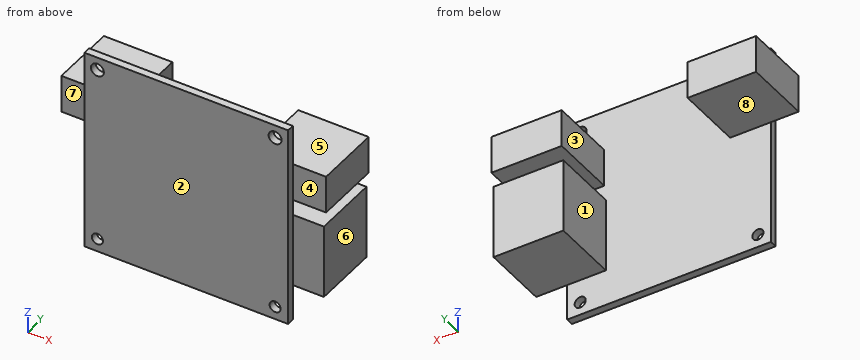
Autodesk Inventor part; units mm, degrees
ref_plane "YZ Plane" through (0, 0, 0) normal (1, 0, 0) x (0, 1, 0)
ref_plane "XZ Plane" through (0, 0, 0) normal (0, 1, 0) x (-1, 0, 0)
ref_plane "XY Plane" through (0, 0, 0) normal (0, 0, 1) x (1, 0, 0)
sketch "Sketch1" plane through (0, 0, 0) normal (0, 1, 0) x (-1, 0, 0)
  line L0 (0, 0) -> (-55, 0)
  line L1 (-55, 0) -> (-55, -55)
  line L2 (-55, -55) -> (0, -55)
  line L3 (0, -55) -> (0, 0)
  circle A0 centre (-3.5, -51.5) radius 1.5
  circle A1 centre (-51.5, -51.5) radius 1.5
  circle A2 centre (-3.5, -3.5) radius 1.75
  circle A3 centre (-51.5, -3.5) radius 1.75
  line L4 (-80.9711, 26.8887) -> (29.0289, 26.8887) construction
  line L5 (29.0289, 26.8887) -> (29.0289, -83.1113) construction
  line L6 (29.0289, -83.1113) -> (-80.9711, -83.1113) construction
  line L7 (-80.9711, -83.1113) -> (-80.9711, 26.8887) construction
  dimension "d1" = 55
  dimension "d4" = 55
  dimension "d49" = 3.5
  dimension "d50" = 3.5
  dimension "d51" = 3
  dimension "d54" = 3
  dimension "d55" = 3.5
  dimension "d56" = 3.5
  dimension "d59" = 3.5
  dimension "d60" = 3.5
  dimension "d61" = 3.5
  dimension "d62" = 3.5
  dimension "d63" = 3.5
  dimension "d64" = 3.5
  dimension "d90" = 110
extrude "Extrusion1" add sketch "Sketch1" along normal blind 2
sketch "Sketch4" plane through (0, 2, 0) normal (0, 1, 0) x (1, 0, 0)
  line L0 (-26.0558, 81.8781) -> (83.9442, 81.8781) construction
  line L1 (83.9442, 81.8781) -> (83.9442, -28.1219) construction
  line L2 (83.9442, -28.1219) -> (-26.0558, -28.1219) construction
  line L3 (-26.0558, -28.1219) -> (-26.0558, 81.8781) construction
  point P0 (0, 0)
  dimension "d77" = 110
sketch "Sketch5" plane through (0, 2, 0) normal (0, 1, 0) x (1, 0, 0)
  line L0 (44.5715, 45.2054) -> (63.4108, 45.2054)
  line L1 (63.4108, 45.2054) -> (63.4108, 25.2259)
  line L2 (63.4108, 25.2259) -> (44.5715, 25.2259)
  line L3 (44.5715, 25.2259) -> (44.5715, 45.2054)
  line L4 (45, 21) -> (64, 21)
  line L5 (64, 21) -> (64, 10.8389)
  line L6 (64, 10.8389) -> (45, 10.8389)
  line L7 (45, 10.8389) -> (45, 21)
  line L8 (-7.4993, 21) -> (11, 21)
  line L9 (11, 21) -> (11, 10.8389)
  line L10 (11, 10.8389) -> (-7.4993, 10.8389)
  line L11 (-7.4993, 10.8389) -> (-7.4993, 21)
  point P0 (0, 0)
extrude "Extrusion2" add sketch "Sketch5" along normal blind 18
properties part number "motorcontroller"
Input: part model. Units: mm. Frame: model coordinates. Face numbers are marked on the shaded views. A direction names the side the tool comes from. Give positions to 0.01 mm unless a question says otherwise; leave off trailing zeros. Order: outer loops, then holes, each group sorted by start corner. A loop starts at its lowest first (then second) coordinate and runs counter-clockwise, first axis right, second up. Notation, with made-up numbers: (15.5, 52) - (21.5, 52) arc R26 cw to (21.5, 75) - close; hole circle Ø10 at (72, -16.5). An arc over 180 degrees is marked (long way). One line per item, written item: value.
1. Cut plane D-D, the plane z = -38.5. Output: boundary loops of the cut face in (x, y).
Determined:
outline: (0, 0) - (55, 0) - (55, 2) - (63.41, 2) - (63.41, 20) - (44.57, 20) - (44.57, 2) - (0, 2) - close
2. Reachability of the marked faces 4, 5, 6, 7 and 8 from +Z, -Z, +X, -X, +Y, -Y: full face, straight path, thin tool, end or side. Return the list, or none.
Determined:
face 4: +Z, -Z, +X, -Y
face 5: +Z, +X, -X, +Y
face 6: -Z, +X, +Y, -Y
face 7: +Z, -Z, -X, -Y
face 8: -Z, +X, -X, +Y
3. Pin query (flat end, axial travel): pin 1 Ø2 at (x, z) = (1, -25) entering from +Y; pin 2 Ø5.5 at (x, y) = (50, 9.5) entering from +Z; pin 3 Ø9 at (y, z) = (9.5, -38.5) entering from -X; pin 4 Ø3 at (x, z) = (51.5, -3.5) entering from -Y. Return the tip coordinate at first contact, or that it passes through.
Determined:
pin 1: y = 2
pin 2: z = -10.84
pin 3: x = 44.57
pin 4: through
4. Cut plane A-A, the plane y = 18.5. Output: boundary loops of the cut face in (x, z), and give its area (3 significant figures).
Determined:
outline: (-7.5, -21) - (11, -21) - (11, -10.84) - (-7.5, -10.84) - close; (44.57, -45.21) - (63.41, -45.21) - (63.41, -25.23) - (44.57, -25.23) - close; (45, -21) - (64, -21) - (64, -10.84) - (45, -10.84) - close
area: 757 mm2
5. Cut plane C-C, the plane x = 3.5. Output: boundary loops of the cut face in (y, z).
Determined:
outline: (0, -55) - (2, -55) - (2, -53) - (0, -53) - close; (0, -50) - (2, -50) - (2, -21) - (20, -21) - (20, -10.84) - (2, -10.84) - (2, -5.25) - (0, -5.25) - close; (0, -1.75) - (2, -1.75) - (2, 0) - (0, 0) - close
6. Cut plane B-B, the plane z = -51.5. Output: boundary loops of the cut face in (x, y).
Determined:
outline: (0, 0) - (2, 0) - (2, 2) - (0, 2) - close; (5, 0) - (50, 0) - (50, 2) - (5, 2) - close; (53, 0) - (55, 0) - (55, 2) - (53, 2) - close
7. Line query: probe 1 along Z at (x, y) = (3.5, 1.6); probe 2 along Z at (x, y) = (54, 7.75); probe 3 along X at (y, z) = (12.5, -15). Output: solid intervals per line, ascending.
Determined:
probe 1: -55 to -53, -50 to -5.25, -1.75 to 0
probe 2: -45.21 to -25.23, -21 to -10.84
probe 3: -7.5 to 11, 45 to 64
8. Draft query along X for the marked faces 1, 2 and 3. Return one class per face: released by +X, released by -X, zero draft, split by the parting line, or undercut.
Determined:
face 1: released by -X
face 2: zero draft
face 3: undercut
